from build123d import *

# Parameters (mm, degrees)
BOSS_EXTRUDE1_DEPTH = 8.95
SKETCH1_3_R         = 4.95
BOSS_EXTRUDE2_DEPTH = 5


with BuildPart() as part:
    # Sketch1 → Boss-Extrude1 (new body)
    with BuildSketch(Plane(origin=(0, 0, 0), x_dir=(1, 0, 0), z_dir=(0, 1, 0))):
        Polygon((2.309401077, 4), (-2.309401077, 4), (-4.618802154, 0), (-2.309401077, -4), (2.309401077, -4), (4.618802154, 0), align=None)
        with BuildLine():
            Line((-1.757128339, 2.05), (1.757128339, 2.05))
            ThreePointArc((1.757128339, 2.05), (2.7, 0), (1.757128339, -2.05))
            Line((1.757128339, -2.05), (-1.757128339, -2.05))
            ThreePointArc((-1.757128339, -2.05), (-2.7, 0), (-1.757128339, 2.05))
        make_face(mode=Mode.SUBTRACT)
    extrude(amount=BOSS_EXTRUDE1_DEPTH)

    # Sketch1_3 → Boss-Extrude2 (add)
    with BuildSketch(Plane(origin=(0, 0, 0), x_dir=(1, 0, 0), z_dir=(0, 1, 0))):
        Circle(SKETCH1_3_R)
        Polygon((4.618802154, 0), (2.309401077, 4), (-2.309401077, 4), (-4.618802154, 0), (-2.309401077, -4), (2.309401077, -4), align=None, mode=Mode.SUBTRACT)
        Polygon((2.309401077, -4), (4.618802154, 0), (2.309401077, 4), (-2.309401077, 4), (-4.618802154, 0), (-2.309401077, -4), align=None)
        with BuildLine():
            ThreePointArc((1.757128339, -2.05), (2.7, 0), (1.757128339, 2.05))
            Line((1.757128339, 2.05), (-1.757128339, 2.05))
            ThreePointArc((-1.757128339, 2.05), (-2.7, 0), (-1.757128339, -2.05))
            Line((-1.757128339, -2.05), (1.757128339, -2.05))
        make_face(mode=Mode.SUBTRACT)
    extrude(amount=-BOSS_EXTRUDE2_DEPTH)


solid = part.part
For this review, take the finished solid that the model builds, in its own axes (mm). A direction names the side the tool comes from. Round coordinates to 2 decimals unless told otherwise and drop trailing zeros. Order: outer loops, then holes, each group sorted by start corner. A loop starts at its lowest first (then second) coordinate and runs counter-clockwise, first axis right, second up. Notation, with made-up numbers: M 20.5,32.25 L 25.5,32.25 A33 ccw 25.5,65.25 Z; hole C 36,71.5 d8. An arc over 180 degrees is marked long. Use a Markdown table: item, result. Add a question column.
Item 1: Add section C-C, the plane z = 1.5. Give the boundary of the cut face in (x, y) (3 decimals).
Item 2: Mouldability with a two-part tool opening along X and no side actions: class faces 5 (the flat face through (-3.48, 4.41, 1.97)), 6 (the flat face through (3.448, 4.412, 2.028)), 7 (the flat face through (-4, 0, 2)), 8 (the flat face through (0, 2, 2.05)) as released by +X, released by -X, zero draft, split by the parting line, or undercut.
Item 3: Tool access review of faces 1 (the flat face through (0, 4, -4)), 2 (the cylindrical face through (2.7, 2.1, 0)), 3 (the flat face through (0, 4, 4)), 4 (the flat face through (3.48, 4.41, -1.97)): name each direction out of +Z, -Z, +X, -X, +Y, -Y from which nothing blocks a thin tool from reaching the whole face with its end or side.
Item 4: Add section D-D, the plane x = -3.25. Give the boundary of the cut face in (y, z).
Item 5: Add section A-A, the plane x = 0. Give the boundary of the cut face in (y, z), then the cut area to 3 significant figures.
Item 6: Add section B-B, the plane y = 7. Give the boundary of the cut face in (x, z).
Item 7: Insertion check: pin 1 (2.5 mm diameter, centred on x = 0, y = 2.5, fed in from +Z); pin 2 (1.5 mm diameter, centred on x = 3.5, y = -0.5, fed in from +Z); pin 3 (3 mm diameter, centred on y = 3, z = 1, fed in from -X). Each pin has a flat end and moves straight along its axis. Give the tip position at first contact, or say it passes through.
Item 8: To check wall thickness, follow line 1 along Z through (x, y) = (0.75, 5.25); line 2 along Z through (x, y) = (2, 6.5); line 3 along X through (y, z) = (-0.75, -0.5). State the ranges of each line that lie inside material, in increasing order.
Geometry results:
| question | item | result |
|---|---|---|
| 1 | outline | M -4.717,-5 L -2.245,-5 L -2.245,8.95 L -3.753,8.95 L -3.753,0 L -4.717,0 Z; M 2.245,-5 L 4.717,-5 L 4.717,0 L 3.753,0 L 3.753,8.95 L 2.245,8.95 Z |
| 2 | face 5 | released by -X |
| 2 | face 6 | released by +X |
| 2 | face 7 | zero draft |
| 2 | face 8 | undercut |
| 3 | face 1 | -Z, +X, -X, +Y |
| 3 | face 2 | +Y, -Y |
| 3 | face 3 | +Z, +X, -X, +Y |
| 3 | face 4 | -Z, +X, +Y |
| 4 | outline | M -5,-3.73 L 0,-3.73 L 0,-2.37 L 8.95,-2.37 L 8.95,2.37 L 0,2.37 L 0,3.73 L -5,3.73 Z |
| 5 | outline | M -5,-4.95 L 0,-4.95 L 0,-4 L 8.95,-4 L 8.95,-2.05 L -5,-2.05 Z; M -5,2.05 L 8.95,2.05 L 8.95,4 L 0,4 L 0,4.95 L -5,4.95 Z |
| 5 | area | 63.9 mm² |
| 6 | outline | M -4.62,0 L -2.31,-4 L 2.31,-4 L 4.62,0 L 2.31,4 L -2.31,4 Z; hole M -1.76,-2.05 L 1.76,-2.05 A2.7 ccw 1.76,2.05 L -1.76,2.05 A2.7 ccw Z |
| 7 | pin 1 | stops at z = 4 |
| 7 | pin 2 | stops at z = 4.12 |
| 7 | pin 3 | stops at x = -4.62 |
| 8 | line 1 | z = -4 to -2.05, 2.05 to 4 |
| 8 | line 2 | z = -4 to -1.81, 1.81 to 4 |
| 8 | line 3 | x = -4.92 to -2.65, 2.65 to 4.92 |
